Design review of the part built by this model. Coordinates are the model's own, in mm. A direction names the side the tool comes from. Coordinates: 2 decimals unless noted, no trailing zeros. Write each loop counter-clockwise with the first axis right and the second up, starting at its lowest first coordinate (ties: lowest second). Pieces come first, ordered by that corner, then holes.
Q1. For probe 1 along X at (y, z) = (2, -10); probe 2 along Z at (x, y) = (-13, 3.5); probe 3 along Z at (x, y) = (16, 7.25), list the stretches that pass through material, from the lowest coordinate up.
Q2. Take a section at A-A (y = 6). Give the boundary of the cut face in (x, z).
Q3. Mouldability with a two-part tool opening along Z and no side actions: class faces 5 (the flat face through (14, 4, -4)), 6 (the flat face through (17.32, 3.94, 2.03)), 7 (the cylindrical face through (16.837, 3.944, -0.195)), 8 (the flat face through (0, 8, 0)) as pulls with the +Z half, pulls with the -Z half, needs draft (parallel to the pull), parting line crosses it, or undercut.
Q4. Machinability: for faces 1 (the flat face through (12.5, 4, -8)), 2 (the flat face through (14, 4, 4)), 3 (the flat face through (-12.5, 4, -8)), 4 (the flat face through (-14, 4, 4)), which of the approach directions +Z, -Z, +X, -X, +Y, -Y give a long, thin tool a straight path to every point of the face, cutting with its end or side? Answer none if there is none.
Q5. Insertion check: pin 1 (4 mm diameter, centred on y = 2.5, z = 6.5, fed in from +X); pin 2 (0.9 mm diameter, centred on x = -14, y = 5.5, fed in from +Z); pin 3 (3 mm diameter, centred on y = 2, z = 3, fed in from -X). Each pin has a flat end and moves straight along its axis. Give the tip position at first contact, or say it passes through.
Q6. Take a section at B-B (z = 5.5). Give the boundary of the cut face in (x, y), and give its area (3 significant figures).
```python
from build123d import *

# Parameters (mm, degrees)
SKETCH_1_R           = 1.5
F_8MM_DEPTH          = 8
MOVE_FACE_25_23_BY   = 1
MOVE_FACE_25_23_2_BY = 1


with BuildPart() as part:
    # 草图1 → 外壳模块组合包络_厚度暂估8mm (new body)
    with BuildSketch(Plane(origin=(0, 0, 0), x_dir=(1, 0, 0), z_dir=(0, 1, 0))):
        Polygon((-19.35, 0), (-15.35, -4), (-12.5, -4), (-12.5, -12.5), (12.5, -12.5), (12.5, -4), (15.35, -4), (19.35, 0), (15.35, 4), (12.5, 4), (12.5, 12.5), (-12.5, 12.5), (-12.5, 4), (-15.35, 4), align=None)
        with Locations(Location((-15.35, 0, 0), (0, 0, 270))):
            Circle(SKETCH_1_R, mode=Mode.SUBTRACT)
        with Locations(Location((15.35, 0, 0), (0, 0, 270))):
            Circle(SKETCH_1_R, mode=Mode.SUBTRACT)
    extrude(amount=F_8MM_DEPTH)

    # Move Face 25_23: a face moved inward by 1.0
    extrude(part.faces().sort_by_distance((0, 4, -12.5))[0], amount=MOVE_FACE_25_23_BY, dir=(0, 0, 1), mode=Mode.SUBTRACT)

    # Move Face 25_23 2: a face moved inward by 1.0
    extrude(part.faces().sort_by_distance((0, 4, 12.5))[0], amount=MOVE_FACE_25_23_2_BY, dir=(0, 0, -1), mode=Mode.SUBTRACT)


solid = part.part
```
Response:
1. probe 1: x = -12.5 to 12.5
1. probe 2: z = -4 to 4
1. probe 3: z = -3.35 to -1.35, 1.35 to 3.35
2. outline: (-19.35, 0) - (-15.35, -4) - (-12.5, -4) - (-12.5, -11.5) - (12.5, -11.5) - (12.5, -4) - (15.35, -4) - (19.35, 0) - (15.35, 4) - (12.5, 4) - (12.5, 11.5) - (-12.5, 11.5) - (-12.5, 4) - (-15.35, 4) - close; hole circle Ø3 at (-15.35, 0); hole circle Ø3 at (15.35, 0)
3. face 5: pulls with the -Z half
3. face 6: pulls with the +Z half
3. face 7: undercut
3. face 8: needs draft
4. face 1: -Z, +X, +Y, -Y
4. face 2: +Z, +X, +Y, -Y
4. face 3: -Z, -X, +Y, -Y
4. face 4: +Z, -X, +Y, -Y
5. pin 1: stops at x = 12.5
5. pin 2: stops at z = 4
5. pin 3: stops at x = -17.85
6. outline: (-12.5, 0) - (12.5, 0) - (12.5, 8) - (-12.5, 8) - close
6. area: 200 mm2
